Study the drawing (mm; zero at the part's minimum x, y, z) and answer. A direction names the side the tool comes from. Round coordinates to 2 decimals unless told otherwise and drop trailing zeros. Answer in a Markdown table with one row per item. Add a question column.
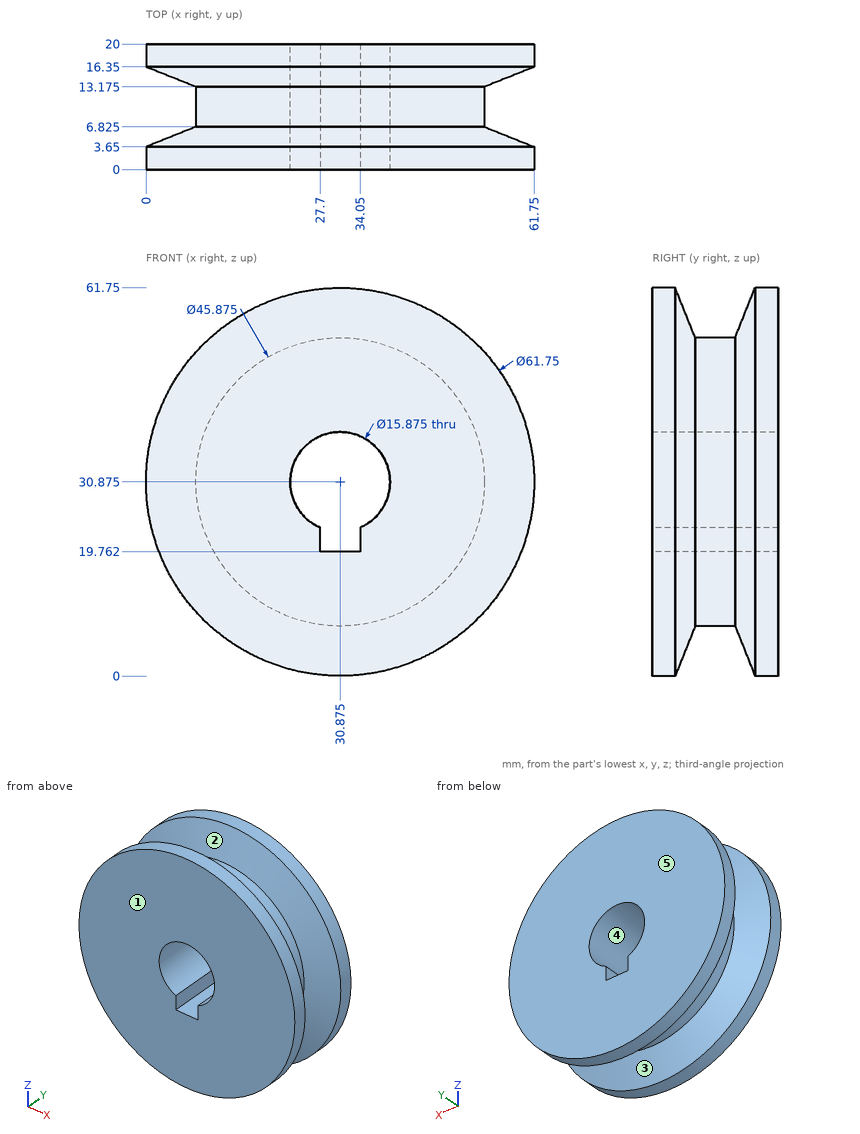
Item 1: Consider L1, parallel to X at y = 1, z = 31.5; L2, parallel to X at y = 8.25, z = 31.5 (1 decimal); L3, parallel to Z at x = 41, y = 11.25 (1 decimal). Determine where each line is inside the solid, lowest interval first. Write a range as from..to.
Item 2: The mould has two halves that part along Z. Classify the marked faces 3, 4 and 5: +Z half, -Z half, draft (parallel to the pull), parting line (faces both ways), or undercut.
Item 3: Flat-ended cylindrical pins translate along their axes: P1, Ø12, axis at x = 39, y = 11, coming from the +Z side; P2, Ø3, axis at y = 9.5, z = 21, coming from the -X side; P3, Ø8, axis at x = 20, y = 5, coming from the -Z side. Find the tip coordinate at first contact, or state that the pin passes through.
Item 4: For the marked faces 1 and 2, determine the directions among +Z, -Z, +X, -X, +Y, -Y from which every point of the face is accessible in a straight line to the end or side of a thin tool.
Here are the results:
| question | item | result |
|---|---|---|
| 1 | L1 | x = 0.01..22.96, 38.79..61.74 |
| 1 | L2 | x = 7.9..23, 38.8..53.8 |
| 1 | L3 | z = 10.3..51.5 |
| 2 | face 3 | parting line |
| 2 | face 4 | undercut |
| 2 | face 5 | draft |
| 3 | P1 | stops at z = 61.27 |
| 3 | P2 | stops at x = 9.52 |
| 3 | P3 | stops at z = 0.83 |
| 4 | face 1 | +Z, -Z, +X, -X, -Y |
| 4 | face 2 | none |
